Part print with two shaded views. Sizes in mm from the minimum x, y, z corner. Give positions to 0.01 mm unless a question says otherwise; leave off trailing zeros. Write each loop counter-clockwise with the first axis right and the second up, starting at its lowest first coordinate (ties: lowest second). Pieces come first, ordered by that corner, then holes. Notation, with made-up numbers: (38, -3) -> (95, -3) arc R30 cw to (95, 25) -> close; hole circle Ø10 at (24.25, 38). An arc over 180 degrees is marked (long way). Answer as a JSON object with one key per item and string values.
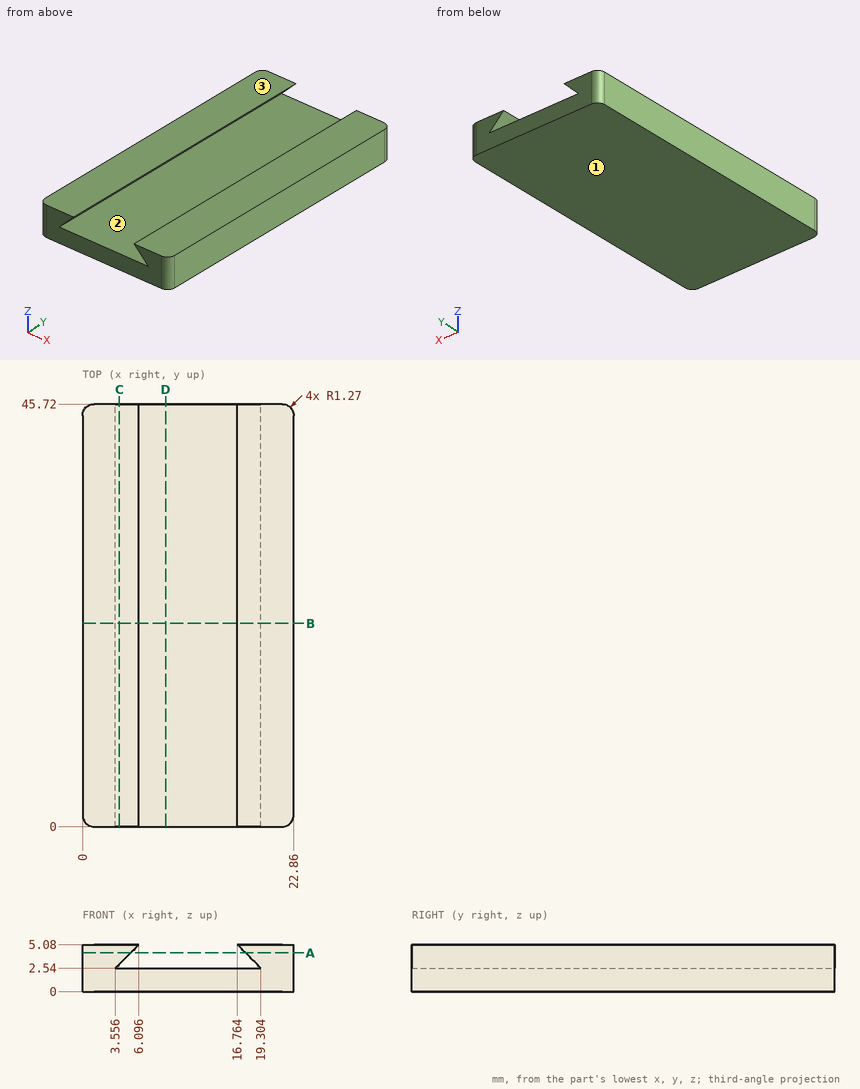
1) Wall check: probe 1 along Z at (x, y) = (13.25, 40); probe 2 along Z at (x, y) = (5, 39); probe 3 along X at (y, z) = (26, 3.8). Give the ranges that are in metal, low to high.
Model answer:
{"probe 1": "z = 0 to 2.54", "probe 2": "z = 0 to 2.54, 3.98 to 5.08", "probe 3": "x = 0 to 4.82, 18.04 to 22.86"}
2) Slice it at D-D (x = 9). List the corners of the cut face in (y, z).
Model answer:
{"outline": "(0, 0) -> (45.72, 0) -> (45.72, 2.54) -> (0, 2.54) -> close"}
3) Slice it at B-B (y = 22). List the corners of the cut face in (x, z).
Model answer:
{"outline": "(0, 0) -> (22.86, 0) -> (22.86, 5.08) -> (16.76, 5.08) -> (19.3, 2.54) -> (3.56, 2.54) -> (6.1, 5.08) -> (0, 5.08) -> close"}
4) Slice it at C-C (x = 4). List the corners of the cut face in (y, z), then the cut area to 3 significant figures.
Model answer:
{"outline": "(0, 0) -> (45.72, 0) -> (45.72, 2.54) -> (0, 2.54) -> close; (0, 2.98) -> (45.72, 2.98) -> (45.72, 5.08) -> (0, 5.08) -> close", "area": "212 mm2"}
5) Mould opens along Z. For the marked faces 1, 2 and 3 say: released by +Z, released by -Z, zero draft, split by the parting line, or undercut.
Model answer:
{"face 1": "released by -Z", "face 2": "undercut", "face 3": "released by +Z"}
6) Slice it at A-A (z = 4.2). List the corners of the cut face in (x, y), then the cut area to 3 significant figures.
Model answer:
{"outline": "(0, 1.27) arc R1.27 ccw to (1.27, 0) -> (5.22, 0) -> (5.22, 45.72) -> (1.27, 45.72) arc R1.27 ccw to (0, 44.45) -> close; (17.64, 0) -> (21.59, 0) arc R1.27 ccw to (22.86, 1.27) -> (22.86, 44.45) arc R1.27 ccw to (21.59, 45.72) -> (17.64, 45.72) -> close", "area": "476 mm2"}
